Check sheet for the modelled part. Datum: model origin and axes. Units: mm. Face numbers are marked on the shaded views. A direction names the side the tool comes from. Round coordinates to 2 decimals unless told otherwise and drop trailing zeros. Loops run counter-clockwise (first coordinate to the right, second up) from the corner with the lowest first, then second, coordinate; pieces in that order, holes last. Notation, with made-up numbers: (21.25, -4) - (52.25, -4) arc R29 cw to (52.25, 23) - close; hole circle Ø4 at (-40, 59). An arc over 180 degrees is marked (long way). Put each result on its own line as item: value. Start each with the question number.
Item 1: Section check A-A, the plane x = 5.5. Record the cut outline in (y, z), and give its area (3 significant figures).
Item 2: Gauge pin test, flat ends, axial feed: pin 1 Ø5 at (x, z) = (-11, 3) entering from -Y; pin 2 Ø2.5 at (x, z) = (1.5, 5) entering from +Y; pin 3 Ø4 at (y, z) = (1, 7.5) entering from +X. Record the tip position at first contact, or that the pin passes through.
Item 3: Tool access check on the marked faces 5, 6, 7, 8 and 9. Record the directions out of +Z, -Z, +X, -X, +Y, -Y that give a thin tool (end or side, any length) a straight path to the whole face; none if there is none.
Item 4: Section check B-B, the plane y = 13.5. Record the cut outline in (x, z).
Item 5: Material ranges on line 1 along X through (y, z) = (6, 5); line 2 along X through (y, z) = (-6, 0.75); line 3 along Y through (x, z) = (10.5, 4), recorded low to high.
Item 6: Section check C-C, the plane x = -0.5. Record the cut outline in (y, z).
Item 7: Draft check along Y on the marked faces 1, 2, 3 and 4. Enter one of: pulls with the +Y half, pulls with the -Y half, needs draft (parallel to the pull), parting line crosses it, or undercut.
Item 8: Section check D-D, the plane z = 8. Give the number of separate pieces and of enclosed holes in the cut face, and give its area (3 significant figures).
from build123d import *

# Parameters (mm, degrees)
SKETCH_1_R      = 1.6
EXTRUDE_1_DEPTH = 9
FILLET_1_R      = 2
SKETCH_2_R      = 4
SKETCH_2_R_2    = 2
EXTRUDE_2_DEPTH = 9
FILLET_2_R      = 3


with BuildPart() as part:
    # 草图1 → 凸台-拉伸1 (new body)
    with BuildSketch(Plane.XY):
        Polygon((0, 19.5), (-16.887495374, -9.75), (16.887495374, -9.75), align=None)
        with Locations((0, 13.5)):
            Circle(SKETCH_1_R, mode=Mode.SUBTRACT)
        with Locations((11.691342951, -6.75)):
            Circle(SKETCH_1_R, mode=Mode.SUBTRACT)
        with Locations((-11.691342951, -6.75)):
            Circle(SKETCH_1_R, mode=Mode.SUBTRACT)
        Polygon((8.227241336, -4.75), (0, 9.5), (-8.227241336, -4.75), align=None, mode=Mode.SUBTRACT)
    extrude(amount=EXTRUDE_1_DEPTH)

    # 圆角1
    fillet_1_edges = [part.edges().sort_by_distance(p)[0] for p in [
        (-8.227241336, -4.75, 4.5),
        (8.227241336, -4.75, 4.5),
        (0, 9.5, 4.5),
        (16.887495374, -9.75, 4.5),
        (-16.887495374, -9.75, 4.5),
        (0, 19.5, 4.5),
    ]]
    fillet(fillet_1_edges, radius=FILLET_1_R)

    # 草图2 → 凸台-拉伸2 (add)
    # profile 1 of 3: a face of its own
    with BuildSketch(Plane.XY.offset(9)):
        with Locations((10.522208656, 6.075)):
            Circle(SKETCH_2_R)
        with Locations((10.522208656, 6.075)):
            Circle(SKETCH_2_R_2, mode=Mode.SUBTRACT)
    # profile 2 of 3: a face of its own
    with BuildSketch(Plane.XY.offset(9)):
        with Locations((-10.522208656, 6.075)):
            Circle(SKETCH_2_R)
        with Locations((-10.522208656, 6.075)):
            Circle(SKETCH_2_R_2, mode=Mode.SUBTRACT)
    # profile 3 of 3: a face of its own
    with BuildSketch(Plane.XY.offset(9)):
        with Locations((0, -12.15)):
            Circle(SKETCH_2_R)
        with Locations((0, -12.15)):
            Circle(SKETCH_2_R_2, mode=Mode.SUBTRACT)
    extrude(amount=-EXTRUDE_2_DEPTH)

    # 圆角2
    fillet_2_edges = [part.edges().sort_by_distance(p)[0] for p in [
        (3.2, -9.75, 4.5),
        (-3.2, -9.75, 4.5),
        (6.843747687, 7.646281292, 4.5),
        (10.043747687, 2.103718708, 4.5),
        (-10.043747687, 2.103718708, 4.5),
        (-6.843747687, 7.646281292, 4.5),
    ]]
    fillet(fillet_2_edges, radius=FILLET_2_R)


solid = part.part
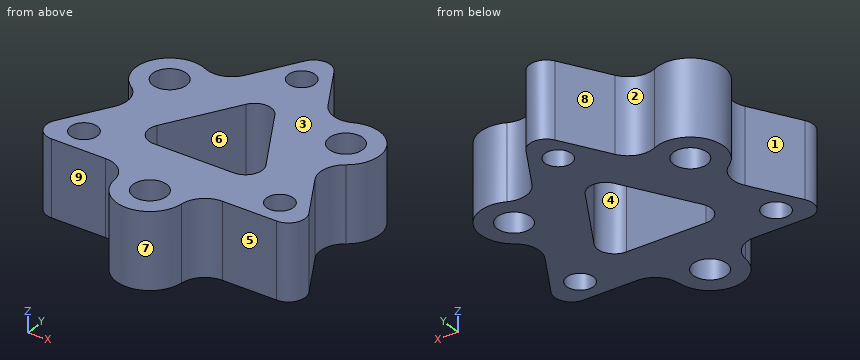
Check result:
1. outline: (-10.14, 0) - (-4.61, 0) - (-4.61, 9) - (-10.14, 9) - close; (-0.03, 0) - (10.23, 0) - (10.23, 9) - (-0.03, 9) - close
1. area: 142 mm²
2. pin 1: y = -9.75
2. pin 2: y = 17.48
2. pin 3: x = 13.08
3. face 5: +Z, -Z, +X, -Y
3. face 6: +Z, -Z
3. face 7: +Z, -Z, -Y
3. face 8: +Z, -Z, -X, +Y
3. face 9: +Z, -Z, -X, -Y
4. outline: (-3.46, 0) - (-1.6, 0) - (-1.6, 9) - (-3.46, 9) - close; (1.6, 0) - (3.46, 0) - (3.46, 9) - (1.6, 9) - close
5. line 1: -14.52 to -12.52, -8.52 to -2.02, 2.02 to 8.52, 12.52 to 14.52
5. line 2: -14.72 to -13.1, -10.28 to 10.28, 13.1 to 14.72
5. line 3: -9.75 to -7.82, -5.68 to 4.08, 8.07 to 10.07
6. outline: (-16.12, 0) - (-14.09, 0) - (-14.09, 9) - (-16.12, 9) - close; (-10.21, 0) - (-4.75, 0) - (-4.75, 9) - (-10.21, 9) - close; (7.44, 0) - (11.98, 0) - (11.98, 9) - (7.44, 9) - close; (15.02, 0) - (17.44, 0) - (17.44, 9) - (15.02, 9) - close
7. face 1: undercut
7. face 2: pulls with the +Y half
7. face 3: needs draft
7. face 4: undercut
8. separate pieces: 1
8. enclosed holes: 7
8. area: 459 mm²
